```python
from build123d import *

# Parameters (mm, degrees)
SKETCH1_W           = 19.9898
SKETCH1_H           = 27.94
BOSS_EXTRUDE1_DEPTH = 4.318
SKETCH2_W           = 19.9898
SKETCH2_H           = 27.94
BOSS_EXTRUDE2_DEPTH = 4.318
SKETCH3_R           = 2.9972
CUT_EXTRUDE3_DEPTH  = 5.318
SKETCH4_R           = 2.9972
CUT_EXTRUDE4_DEPTH  = 5.318


with BuildPart() as part:
    # Sketch1 → Boss-Extrude1 (new body)
    with BuildSketch(Plane(origin=(0, 0, 0), x_dir=(1, 0, 0), z_dir=(0, 1, 0))):
        with Locations((9.9949, 13.97)):
            Rectangle(SKETCH1_W, SKETCH1_H)
    extrude(amount=BOSS_EXTRUDE1_DEPTH)

    # Sketch2 → Boss-Extrude2 (add)
    with BuildSketch(Plane(origin=(0, 0, -27.94), x_dir=(-1, 0, 0), z_dir=(0, 0, -1))):
        with Locations((-9.9949, 13.97)):
            Rectangle(SKETCH2_W, SKETCH2_H)
    extrude(amount=-BOSS_EXTRUDE2_DEPTH)

    # Sketch3 → Cut-Extrude3 (cut, through all)
    with BuildSketch(Plane(origin=(0, 4.318, 0), x_dir=(1, 0, 0), z_dir=(0, 1, 0))):
        with Locations((9.9949, 13.97)):
            Circle(SKETCH3_R)
    extrude(amount=-CUT_EXTRUDE3_DEPTH, mode=Mode.SUBTRACT)

    # Sketch4 → Cut-Extrude4 (cut, through all)
    with BuildSketch(Plane.XY.offset(-23.622)):
        with Locations((9.9949, 13.97)):
            Circle(SKETCH4_R)
    extrude(amount=-CUT_EXTRUDE4_DEPTH, mode=Mode.SUBTRACT)


solid = part.part
```
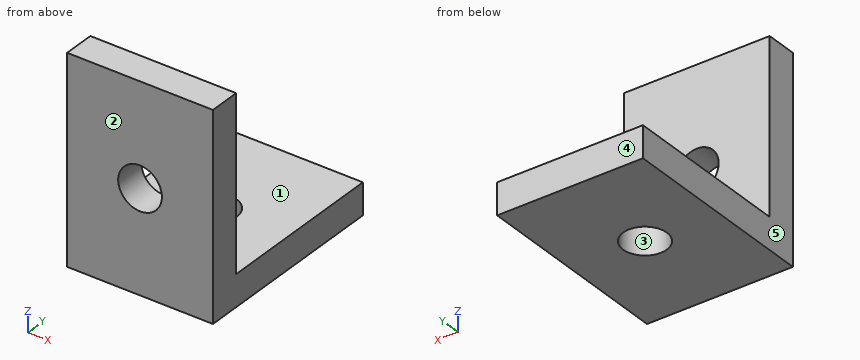
For this review, take the finished solid that the model builds, in its own axes (mm). Face numbers are marked on the shaded views. A direction names the side the tool comes from. Round coordinates to 2 decimals unless told otherwise and drop trailing zeros. Write each loop counter-clockwise with the first axis right and the second up, starting at its lowest first coordinate (ties: lowest second). Pieces come first, ordered by that corner, then holes. Notation, with made-up numbers: (79.5, 44.5) - (120.5, 44.5) arc R30 cw to (120.5, 67.5) - close; hole circle Ø1 at (8, 85). An arc over 180 degrees is marked (long way). Use CSV: the item, a comma, the result in double quotes.
1) Add section A-A on y = 13.97. Write out the cut boundary in (x, z), and give its area (3 significant figures).
Conclusion:
outline,"(0, -27.94) - (7, -27.94) - (7, -23.62) - (0, -23.62) - close; (12.99, -27.94) - (19.99, -27.94) - (19.99, -23.62) - (12.99, -23.62) - close"
area,"60.4 mm^2"
2) Add section B-B on z = -25.25. Write out the cut boundary in (x, y), and give its area (3 significant figures).
Conclusion:
outline,"(0, 0) - (19.99, 0) - (19.99, 27.94) - (0, 27.94) - close; hole circle Ø5.99 at (9.99, 13.97)"
area,"530 mm^2"
3) Add section C-C on x = 8. Write out the cut boundary in (y, z).
Conclusion:
outline,"(0, -27.94) - (11.73, -27.94) - (11.73, -23.62) - (4.32, -23.62) - (4.32, -16.21) - (0, -16.21) - close; (0, -11.73) - (4.32, -11.73) - (4.32, 0) - (0, 0) - close; (16.21, -27.94) - (27.94, -27.94) - (27.94, -23.62) - (16.21, -23.62) - close"
4) The part is to be moulded in two halves that separate along X. For the marked faces 3, 4 and 5, say which applies: pulls with the +X half, pulls with the -X half, needs draft (parallel to the pull), parting line crosses it, or undercut.
Conclusion:
face 3,"undercut"
face 4,"needs draft"
face 5,"pulls with the -X half"
5) Clearance check with flat-ended pins moving along their axes: pin 1 Ø4 at (x, y) = (10.5, 24.5) entering from +Z; pin 2 Ø6 at (x, z) = (14, -13.5) entering from +Y. State where each tip first meets the part, or that it passes through.
Conclusion:
pin 1,"stops at z = -23.62"
pin 2,"stops at y = 4.32"
6) Add section D-D on z = -13.97. Write out the cut boundary in (x, y).
Conclusion:
outline,"(0, 0) - (7, 0) - (7, 4.32) - (0, 4.32) - close; (12.99, 0) - (19.99, 0) - (19.99, 4.32) - (12.99, 4.32) - close"
7) For the marked faces 1 and 2, list the 3-axis set-ups (+Z, -Z, +X, -X, +Y, -Y) from which the entire face can be reached by the end or side of a thin tool; tool diameter is ignored.
Conclusion:
face 1,"+Z, +X, -X, +Y"
face 2,"+Z, -Z, +X, -X, -Y"
8) Wall thickness on line 1 along X through (y, z) = (2.8, -13.97); line 2 along Z through (x, y) = (4, 14); line 3 along Y through (x, z) = (10.5, -2.75): over which ranges is each line inside the solid? List them lowest first. Write a range as from..to.
Conclusion:
line 1,"x = 0..7, 12.99..19.99"
line 2,"z = -27.94..-23.62"
line 3,"y = 0..4.32"
